Build history of the part. All positions in model axes, mm. Face numbers are marked on the shaded views. A direction names the side the tool comes from. Coordinates: 2 decimals unless noted, no trailing zeros. Loops run counter-clockwise (first coordinate to the right, second up) from the corner with the lowest first, then second, coordinate; pieces in that order, holes last.
Item 1: Cut at B-B (z = -1.5). List the corners of the cut face in (x, y) (3 decimals), and give its area (3 significant figures).
Item 2: Drill centre lines: line 1 along X through (y, z) = (9.25, -15) (3 decimals); line 2 along Z through (x, y) = (-6.5, -5.5) (3 decimals); line 3 along Z through (x, y) = (12, -13.75) (3 decimals). Where is each one in solid material? Low to high.
Item 3: Cut at A-A (x = -2). List the corners of the cut face in (y, z) (3 decimals), and give its area (3 significant figures).
Item 4: Mould opens along Z. For the marked faces 1, 2 and 3 say: released by +Z, released by -Z, zero draft, split by the parting line, or undercut.
Item 5: Flat gauge pins, fed straight in: pin 1 (1.5 mm diameter, centred on y = 5.5, z = 6.5, fed in from -X); pin 2 (12 mm diameter, centred on x = 18, z = 3, fed in from +Y) (3 decimals); pin 3 (7.5 mm diameter, centred on x = 20.5, y = 0, fed in from +Z) (3 decimals). Where does each tip first touch, or does it go through?
Item 6: Cut at D-D (x = 15). List the corners of the cut face in (y, z) (3 decimals).
Item 7: Cut at C-C (y = -0.5). List the corners of the cut face in (x, z) (3 decimals).
Item 8: 3-axis set-ups, long thin cutter, end or side, ignore diameter. For the marked faces 4, 5, 6, 7 and 8: which of +Z, -Z, +X, -X, +Y, -Y reach the whole face in a straight line?
from build123d import *

# Parameters (mm, degrees)
F0_W      = 31.75
F0_H      = 9.525
F1_DEPTH  = 3.175
F4_R      = 2.286
F8_R      = 2.286
F10_W     = 55
F10_H     = 25.4
F11_DEPTH = 25.4
F12_W     = 17.5
F12_H     = 21.4
F12_W_2   = 12
F12_H_2   = 23.4
F13_DEPTH = 25.401


with BuildPart() as f1:
    # F0 (on Top) → F1 (new body)
    with BuildSketch(Plane.XY):
        with Locations((15.875, 4.7625)):
            Rectangle(F0_W, F0_H)
    extrude(amount=F1_DEPTH)

    # F5: sweep along a path in F3
    with BuildLine(Plane.YZ.offset(28.575)) as f5_path:
        Line((7.1374, 3.175), (7.1374, 9.525))
        Line((7.1374, 9.525), (11.6275280605, 14.0151280605))
    # F4 (on face) → F5 (sweep)
    with BuildSketch(Plane.XY.offset(3.175)):
        with Locations((28.575, 7.1374)):
            Circle(F4_R)
    sweep(path=f5_path.line, transition=Transition.RIGHT)

    # F9: sweep along a path in F7
    with BuildLine(Plane.YZ.offset(3.175)) as f9_path:
        Line((7.1374, 3.175), (7.1374, 9.525))
        Line((7.1374, 9.525), (11.6275280605, 14.0151280605))
    # F8 (on face) → F9 (sweep)
    with BuildSketch(Plane.XY.offset(3.175)):
        with Locations((3.175, 7.1374)):
            Circle(F8_R)
    sweep(path=f9_path.line, transition=Transition.RIGHT)

    # F10 (on face) → F11 (join)
    with BuildSketch(Plane.XY.offset(3.175)):
        with Locations((15.875, -3.175)):
            Rectangle(F10_W, F10_H)
    extrude(amount=-F11_DEPTH)

    # F12 (on face) → F13 (cut, through all)
    with BuildSketch(Plane(origin=(0, 9.525, 0), x_dir=(-1, 0, 0), z_dir=(0, 1, 0))):
        with Locations((-32.625, -9.525)):
            Rectangle(F12_W, F12_H)
        with Locations((-15.875, -10.525)):
            Rectangle(F12_W_2, F12_H_2)
        with Locations((0.875, -9.525)):
            Rectangle(F12_W, F12_H)
    extrude(amount=-F13_DEPTH, mode=Mode.SUBTRACT)


solid = f1.part
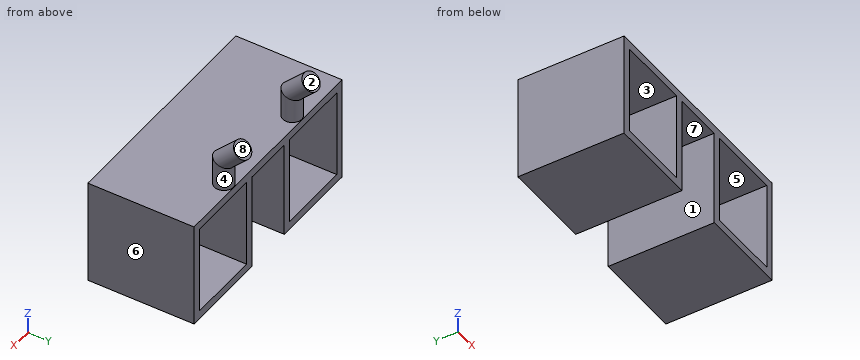
Filled sheet:
1. outline: (-11.625, -15.875) - (-9.625, -15.875) - (-9.625, 9.525) - (-11.625, 9.525) - close; (7.875, -15.875) - (9.875, -15.875) - (9.875, 9.525) - (7.875, 9.525) - close; (21.875, -15.875) - (23.875, -15.875) - (23.875, 9.525) - (21.875, 9.525) - close; (41.375, -15.875) - (43.375, -15.875) - (43.375, 9.525) - (41.375, 9.525) - close
1. area: 203 mm2
2. line 1: x = -11.625 to -9.625, 7.875 to 9.875, 21.875 to 23.875, 41.375 to 43.375
2. line 2: z = -22.225 to -20.225, 1.175 to 3.175
2. line 3: z = 1.175 to 3.175
3. outline: (-15.875, -22.225) - (9.525, -22.225) - (9.525, -20.225) - (-15.875, -20.225) - close; (-15.875, 1.175) - (9.525, 1.175) - (9.525, 3.175) - (-15.875, 3.175) - close
3. area: 102 mm2
4. face 1: zero draft
4. face 2: released by +Z
4. face 3: undercut
5. pin 1: stops at x = 1.07
5. pin 2: stops at y = 9.525
5. pin 3: stops at z = 3.175
6. outline: (-15.875, 1.175) - (9.525, 1.175) - (9.525, 3.175) - (-15.875, 3.175) - close
7. outline: (-11.625, -22.225) - (9.875, -22.225) - (9.875, 1.175) - (21.875, 1.175) - (21.875, -22.225) - (43.375, -22.225) - (43.375, 3.175) - (-11.625, 3.175) - close; hole (-9.625, -20.225) - (7.875, -20.225) - (7.875, 1.175) - (-9.625, 1.175) - close; hole (23.875, -20.225) - (41.375, -20.225) - (41.375, 1.175) - (23.875, 1.175) - close
8. face 4: none
8. face 5: +Y, -Y
8. face 6: +Z, -Z, +X, +Y, -Y
8. face 7: -Z, +Y, -Y
8. face 8: +Z, +X, -X, +Y
